from build123d import *

# Parameters (mm, degrees)
BOSS_EXTRUDE1_DEPTH = 30
CUT_EXTRUDE1_DEPTH  = 13
SKETCH5_R           = 1.5
CUT_EXTRUDE2_DEPTH  = 1
SKETCH6_R           = 1.5
CUT_EXTRUDE3_DEPTH  = 1


with BuildPart() as part:
    # Sketch1 → Boss-Extrude1 (new body)
    with BuildSketch(Plane.XY):
        with BuildLine():
            Line((0, 0), (0, 12))
            Line((0, 12), (10, 12))
            ThreePointArc((10, 12), (16, 6), (22, 12))
            Line((22, 12), (32, 12))
            Line((32, 12), (32, 0))
            Line((32, 0), (0, 0))
        make_face()
    extrude(amount=BOSS_EXTRUDE1_DEPTH)

    # Sketch4 → Cut-Extrude1 (cut, through all)
    with BuildSketch(Plane(origin=(0, 12, 0), x_dir=(1, 0, 0), z_dir=(0, 1, 0))):
        Polygon((5, -2), (3.267949192, -5), (6.732050808, -5), align=None)
        Polygon((5, -28), (6.732050808, -25), (3.267949192, -25), align=None)
        Polygon((29, -28), (30.732050808, -25), (27.267949192, -25), align=None)
        Polygon((29, -2), (27.267949192, -5), (30.732050808, -5), align=None)
    extrude(amount=-CUT_EXTRUDE1_DEPTH, mode=Mode.SUBTRACT)

    # Sketch5 → Cut-Extrude2 (cut)
    with BuildSketch(Plane(origin=(32, 0, 0), x_dir=(0, 0, -1), z_dir=(1, 0, 0))):
        with Locations((-25.5, 7.2)):
            Circle(SKETCH5_R)
        with Locations((-4.5, 7.2)):
            Circle(SKETCH5_R)
    extrude(amount=-CUT_EXTRUDE2_DEPTH, mode=Mode.SUBTRACT)

    # Sketch6 → Cut-Extrude3 (cut)
    with BuildSketch(Plane.ZY):
        with Locations((4.5, 7.661165518)):
            Circle(SKETCH6_R)
        with Locations((25.5, 7.661165518)):
            Circle(SKETCH6_R)
    extrude(amount=-CUT_EXTRUDE3_DEPTH, mode=Mode.SUBTRACT)


solid = part.part
Can you work these out from the model? Positions are in its coordinate system, mm. A direction names the side the tool comes from. Round coordinates to 2 decimals unless told otherwise and drop trailing zeros. Loops run counter-clockwise (first coordinate to the right, second up) from the corner with the lowest first, then second, coordinate; pieces in that order, holes last. Notation, with made-up numbers: (25, -8) - (43, -8) arc R14 cw to (43, 5) - close; hole circle Ø7 at (-30.75, 66). An arc over 180 degrees is marked (long way). Use CSV: the item, a comma, the result in double quotes. Start each with the question number.
1) If we section it at C-C on z = 8.75: Write out the boundary of the cut face in (x, y).
2) For faces 1 (the flat face through (5, 6, 25)), 2 (the flat face through (1, 8, 4)), 3 (the cylindrical face through (31.507, 5.736, 4.825)), which set-ups out of +Z, -Z, +X, -X, +Y, -Y let a thin tool reach every point of the face, with its end or its side?
3) For pin 1 Ø3 at (x, z) = (13.5, 22) entering from +Y; pin 2 Ø0.9 at (y, z) = (7.5, 26) entering from -X; pin 3 Ø2.5 at (y, z) = (7.2, 4.5) entering from +X, each with a flat end and sliding along its axis, tell me the tip position at first contact or that it passes through.
4) If we section it at D-D on z = 4.5: Write out the boundary of the cut face in (x, y), plus the area to 3 significant figures.
5) We'd pull the mould along Y, two halves only. Please class faces 4 (the flat face through (5, 6, 5)), 5 (the cylindrical face through (16, 6, 15)), 6 (the flat face through (1, 8, 25)): released by +Y, released by -Y, zero draft, split by the parting line, or undercut.
6) If we section it at B-B on y = 3.5: Write out the boundary of the cut face in (x, z), plus the area to 3 significant figures.
7) If we section it at A-A on y = 11.25: Write out the boundary of the cut face in (x, z).
8) Please list where these lines run through material, in increasing order: probe 1 along Y at (x, z) = (0.5, 25.5); probe 2 along Y at (x, z) = (31.5, 4.5); probe 3 along Z at (x, y) = (28, 6.25). Write a range as [from, to].
Geometry results:
1,outline,"(0, 0) - (32, 0) - (32, 12) - (22, 12) arc R6 cw to (10, 12) - (0, 12) - close"
2,face 1,"+Y, -Y"
2,face 2,"-X"
2,face 3,"+X"
3,pin 1,"stops at y = 7.53"
3,pin 2,"stops at x = 1"
3,pin 3,"stops at x = 31"
4,outline,"(0, 0) - (3.56, 0) - (3.56, 12) - (0, 12) - (0, 9.16) - (1, 9.16) - (1, 6.16) - (0, 6.16) - close; (6.44, 0) - (27.56, 0) - (27.56, 12) - (22, 12) arc R6 cw to (10, 12) - (6.44, 12) - close; (30.44, 0) - (32, 0) - (32, 5.7) - (31, 5.7) - (31, 8.7) - (32, 8.7) - (32, 12) - (30.44, 12) - close"
4,area,"252 mm2"
5,face 4,"zero draft"
5,face 5,"released by +Y"
5,face 6,"undercut"
6,outline,"(0, 0) - (32, 0) - (32, 30) - (0, 30) - close; hole (3.27, 5) - (5, 2) - (6.73, 5) - close; hole (3.27, 25) - (6.73, 25) - (5, 28) - close; hole (27.27, 5) - (29, 2) - (30.73, 5) - close; hole (27.27, 25) - (30.73, 25) - (29, 28) - close"
6,area,"939 mm2"
7,outline,"(0, 0) - (10.05, 0) - (10.05, 30) - (0, 30) - close; (21.95, 0) - (32, 0) - (32, 30) - (21.95, 30) - close; hole (3.27, 5) - (5, 2) - (6.73, 5) - close; hole (3.27, 25) - (6.73, 25) - (5, 28) - close; hole (27.27, 5) - (29, 2) - (30.73, 5) - close; hole (27.27, 25) - (30.73, 25) - (29, 28) - close"
8,probe 1,"y = [0, 6.16], [9.16, 12]"
8,probe 2,"y = [0, 5.7], [8.7, 12]"
8,probe 3,"z = [0, 3.73], [5, 25], [26.27, 30]"
